Work out the finished part from the listing and answer in its coordinate system (mm). Face numbers are marked on the shaded views. Round coordinates to 2 decimals unless told otherwise and drop trailing zeros. Write each loop counter-clockwise with the first axis right and the second up, starting at its lowest first coordinate (ties: lowest second). Pieces come first, ordered by that corner, then holes.
1. Find section C-C (y = 64). Write down the section's boundary in (x, z), and give its area (3 significant figures).
2. Find section D-D (y = 35.5). Write down the section's boundary in (x, z), and give its area (3 significant figures).
3. Find section B-B (x = 32). Write down the section's boundary in (y, z).
4. Determine the mould class of the marked faces 1 and 2 for opening direction Y: pulls with the +Y half, pulls with the -Y half, needs draft (parallel to the pull), parting line crosses it, or undercut.
5. Find section A-A (z = 4.5). Write down the section's boundary in (x, y).
6. Straight lines are drawn through the part: probe 1 along X at (y, z) = (-76, 10.75); probe 2 along Y at (x, z) = (-28, 2.5); probe 3 along Y at (x, z) = (67.5, 12.1). For each, find the intervals that lie inside material, in ascending order.
7. Flat-ended cylindrical pins translate along their axes: pin 1 Ø12 at (x, y) = (-16, 5) entering from +Z; pin 2 Ø5 at (x, y) = (-67.82, 20.45) entering from -Z. Find the tip coordinate at first contact, or state that the pin passes through.
```python
from build123d import *

# Parameters (mm, degrees)
SCHIZZO1_W                   = 196.27671429
SCHIZZO1_H                   = 160
SCHIZZO1_W_2                 = 160
SCHIZZO1_H_2                 = 146
ESTRUSIONE_ESTRUSIONE1_DEPTH = 10
SCHIZZO2_W                   = 196.27671429
SCHIZZO2_H                   = 160
ESTRUSIONE_ESTRUSIONE2_DEPTH = 4
SCHIZZO3_R                   = 1.5
TAGLIO_ESTRUSIONE1_DEPTH     = 93
SCHIZZO4_R                   = 39
SCHIZZO4_R_2                 = 2.25
SCHIZZO4_R_3                 = 1.5
SCHIZZO4_W                   = 5
SCHIZZO4_H                   = 12
SCHIZZO4_W_2                 = 1.5
SCHIZZO4_H_2                 = 20
TAGLIO_ESTRUSIONE2_DEPTH     = 90


with BuildPart() as part:
    # Schizzo1 → Estrusione-Estrusione1 (new body)
    with BuildSketch(Plane.XY):
        Rectangle(SCHIZZO1_W, SCHIZZO1_H)
        Rectangle(SCHIZZO1_W_2, SCHIZZO1_H_2, mode=Mode.SUBTRACT)
    extrude(amount=ESTRUSIONE_ESTRUSIONE1_DEPTH)

    # Schizzo2 → Estrusione-Estrusione2 (add)
    with BuildSketch(Plane.XY.offset(10)):
        Rectangle(SCHIZZO2_W, SCHIZZO2_H)
    extrude(amount=ESTRUSIONE_ESTRUSIONE2_DEPTH)

    # Schizzo3 → Taglio-Estrusione1 (cut)
    with BuildSketch(Plane(origin=(0, 0, 0), x_dir=(-1, 0, 0), z_dir=(0, 0, -1))):
        with Locations((65.48331215, 76)):
            Circle(SCHIZZO3_R)
        with Locations(Location((-65.48331215, 76, 0), (0, 0, 180))):
            Circle(SCHIZZO3_R)
        with Locations((-65.48331215, -76)):
            Circle(SCHIZZO3_R)
        with Locations(Location((65.48331215, -76, 0), (0, 0, 180))):
            Circle(SCHIZZO3_R)
    extrude(amount=-TAGLIO_ESTRUSIONE1_DEPTH, mode=Mode.SUBTRACT)

    # Schizzo4 → Taglio-Estrusione2 (cut)
    with BuildSketch(Plane(origin=(0, 0, 10), x_dir=(-1, 0, 0), z_dir=(0, 0, -1))):
        with Locations((-32, 0)):
            Circle(SCHIZZO4_R)
        with Locations((3.499999997, 35.499999997)):
            Circle(SCHIZZO4_R_2)
        with Locations((3.499999997, -35.499999997)):
            Circle(SCHIZZO4_R_2)
        with Locations((-67.499999997, 35.499999997)):
            Circle(SCHIZZO4_R_2)
        with Locations((-67.499999997, -35.499999997)):
            Circle(SCHIZZO4_R_2)
        with Locations((41.299094201, 20.449190864)):
            Circle(SCHIZZO4_R_3)
        with Locations((41.299094201, -20.449190864)):
            Circle(SCHIZZO4_R_3)
        with Locations((67.823483409, -20.449190864)):
            Circle(SCHIZZO4_R_3)
        with Locations((67.823483409, 20.449190864)):
            Circle(SCHIZZO4_R_3)
        with Locations((16, 0)):
            Rectangle(SCHIZZO4_W, SCHIZZO4_H)
        with Locations((39.87257761, 0)):
            Rectangle(SCHIZZO4_W_2, SCHIZZO4_H_2)
    extrude(amount=-TAGLIO_ESTRUSIONE2_DEPTH, mode=Mode.SUBTRACT)


solid = part.part
```
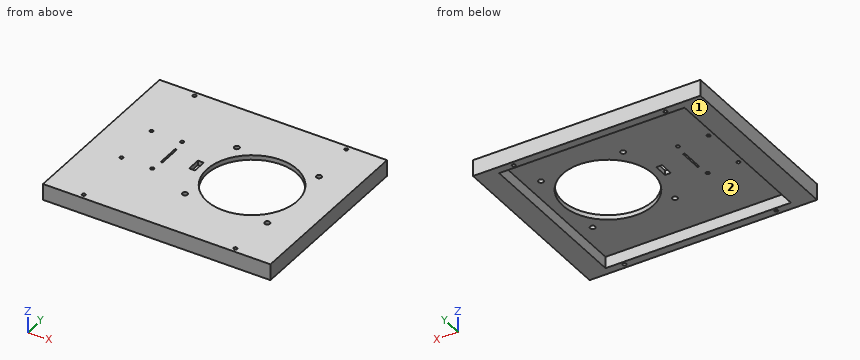
Worked answers:
1. outline: (-98.14, 0) - (-80, 0) - (-80, 10) - (80, 10) - (80, 0) - (98.14, 0) - (98.14, 14) - (-98.14, 14) - close
1. area: 1,150 mm2
2. outline: (-98.14, 0) - (-80, 0) - (-80, 10) - (-5.75, 10) - (-5.75, 14) - (-98.14, 14) - close; (-1.25, 10) - (15.85, 10) - (15.85, 14) - (-1.25, 14) - close; (48.15, 10) - (65.25, 10) - (65.25, 14) - (48.15, 14) - close; (69.75, 10) - (80, 10) - (80, 0) - (98.14, 0) - (98.14, 14) - (69.75, 14) - close
2. area: 983 mm2
3. outline: (-80, 0) - (-73, 0) - (-73, 10) - (-39, 10) - (-39, 14) - (-80, 14) - close; (39, 10) - (73, 10) - (73, 0) - (80, 0) - (80, 14) - (39, 14) - close
4. face 1: needs draft
4. face 2: undercut
5. outline: (-98.14, -80) - (98.14, -80) - (98.14, 80) - (-98.14, 80) - close; hole (-80, -73) - (80, -73) - (80, 73) - (-80, 73) - close; hole circle Ø3 at (-65.48, -76); hole circle Ø3 at (-65.48, 76); hole circle Ø3 at (65.48, -76); hole circle Ø3 at (65.48, 76)
6. probe 1: x = -98.14 to -66.98, -63.98 to 63.98, 66.98 to 98.14
6. probe 2: y = -80 to -73, 73 to 80
6. probe 3: y = -80 to -37.75, -33.25 to -16.15, 16.15 to 33.25, 37.75 to 80
7. pin 1: stops at z = 14
7. pin 2: stops at z = 10
